from build123d import *

# Parameters (mm, degrees)
SKETCH1_W           = 60
SKETCH1_H           = 30
BOSS_EXTRUDE1_DEPTH = 10
FILLET1_R           = 4
SHELL1_T            = -2
SKETCH29_W          = 3
SKETCH29_H          = 10
BOSS_EXTRUDE2_DEPTH = 1
SKETCH30_W          = 2
SKETCH30_H          = 10
BOSS_EXTRUDE3_DEPTH = 1
SKETCH31_W          = 1
SKETCH31_H          = 10
BOSS_EXTRUDE4_DEPTH = 1


with BuildPart() as part:
    # Sketch1 → Boss-Extrude1 (new body)
    with BuildSketch(Plane.XY):
        with Locations((8.508287293, 1.740331492)):
            Rectangle(SKETCH1_W, SKETCH1_H)
    extrude(amount=BOSS_EXTRUDE1_DEPTH)

    # Fillet1
    fillet1_edges = [part.edges().sort_by_distance(p)[0] for p in [
        (-21.491712707, 16.740331492, 5),
        (38.508287293, 16.740331492, 5),
        (38.508287293, -13.259668508, 5),
        (-21.491712707, -13.259668508, 5),
    ]]
    fillet(fillet1_edges, radius=FILLET1_R)

    # Shell1
    shell1_openings = [part.faces().sort_by_distance(p)[0] for p in [
        (8.508287293, 1.740331492, 10),
    ]]
    offset(amount=SHELL1_T, openings=shell1_openings, kind=Kind.INTERSECTION)

    # Sketch29 → Boss-Extrude2 (add)
    with BuildSketch(Plane.XY.offset(2)):
        with Locations((22.008287293, 1.740331492)):
            Rectangle(SKETCH29_W, SKETCH29_H)
        with Locations((8.008287293, 1.740331492)):
            Rectangle(SKETCH29_W, SKETCH29_H)
        with Locations((-5.991712707, 1.740331492)):
            Rectangle(SKETCH29_W, SKETCH29_H)
    extrude(amount=BOSS_EXTRUDE2_DEPTH)

    # Sketch30 → Boss-Extrude3 (add)
    with BuildSketch(Plane.XY.offset(3)):
        with Locations((22.008287293, 1.740331492)):
            Rectangle(SKETCH30_W, SKETCH30_H)
        with Locations((8.008287293, 1.740331492)):
            Rectangle(SKETCH30_W, SKETCH30_H)
        with Locations((-5.991712707, 1.740331492)):
            Rectangle(SKETCH30_W, SKETCH30_H)
    extrude(amount=BOSS_EXTRUDE3_DEPTH)

    # Sketch31 → Boss-Extrude4 (add)
    with BuildSketch(Plane.XY.offset(4)):
        with Locations((22.008287293, 1.740331492)):
            Rectangle(SKETCH31_W, SKETCH31_H)
        with Locations((8.008287293, 1.740331492)):
            Rectangle(SKETCH31_W, SKETCH31_H)
        with Locations((-5.991712707, 1.740331492)):
            Rectangle(SKETCH31_W, SKETCH31_H)
    extrude(amount=BOSS_EXTRUDE4_DEPTH)


solid = part.part
The listing builds one solid part. Answer for the finished solid, in the listing's coordinates (mm). A direction names the side the tool comes from. Round coordinates to 2 decimals unless told otherwise and drop trailing zeros. Order: outer loops, then holes, each group sorted by start corner. A loop starts at its lowest first (then second) coordinate and runs counter-clockwise, first axis right, second up. Notation, with made-up numbers: (-1.5, 83.25) - (44.5, 83.25) arc R18 ccw to (44.5, 92.25) - close; hole circle Ø2 at (85.25, 36). An arc over 180 degrees is marked (long way). Write item = value, one per line. Start each with the question number.
1) Section B-B, the plane y = 11.75 is taken. Write down the section's boundary in (x, z), plus the area to 3 significant figures.
2) For a pull along X with two mould halves and no side action, classify faces 3 (the flat face through (36.508, 2, 6)), 4 (the flat face through (-6, -3.26, 3)), 5 (the flat face through (-21.492, 2, 5)), 6 (the flat face through (6, -12, 10)) as released by +X, released by -X, zero draft, split by the parting line, or undercut.
3) Section C-C, the plane x = -12 is taken. Write down the section's boundary in (y, z), plus the area to 3 significant figures.
4) Section A-A, the plane z = 6.75 is taken. Write down the section's boundary in (x, y).
5) For faces 1 (the flat face through (-6, 6.74, 3)), 2 (the flat face through (8, 16.74, 5)), determine the directions among +Z, -Z, +X, -X, +Y, -Y from which every point of the face is accessible in a straight line to the end or side of a thin tool.
6) Given pin 1 (1.1 mm diameter, centred on x = 22, y = -0.5, fed in from +Z); pin 2 (4 mm diameter, centred on x = 15, y = -9, fed in from +Z), each flat-ended and moving along its own axis, determine where each tip first touches the part or whether it passes through.
7) Straight lines are drawn through the part: L1, parallel to X at y = -2.25, z = 4.75; L2, parallel to X at y = 1, z = 3.5; L3, parallel to Y at x = -12.5, z = 7.25. For each, find the intervals that lie inside material, in ascending order.
Results list:
q1.outline = (-21.49, 0) - (38.51, 0) - (38.51, 10) - (36.51, 10) - (36.51, 2) - (-19.49, 2) - (-19.49, 10) - (-21.49, 10) - close
q1.area = 152 mm^2
q2.face_3 = undercut
q2.face_4 = undercut
q2.face_5 = released by -X
q2.face_6 = zero draft
q3.outline = (-13.26, 0) - (16.74, 0) - (16.74, 10) - (14.74, 10) - (14.74, 2) - (-11.26, 2) - (-11.26, 10) - (-13.26, 10) - close
q3.area = 92.0 mm^2
q4.outline = (-21.49, -9.26) arc R4 ccw to (-17.49, -13.26) - (34.51, -13.26) arc R4 ccw to (38.51, -9.26) - (38.51, 12.74) arc R4 ccw to (34.51, 16.74) - (-17.49, 16.74) arc R4 ccw to (-21.49, 12.74) - close; hole (-19.49, -9.26) arc R2 ccw to (-17.49, -11.26) - (34.51, -11.26) arc R2 ccw to (36.51, -9.26) - (36.51, 12.74) arc R2 ccw to (34.51, 14.74) - (-17.49, 14.74) arc R2 ccw to (-19.49, 12.74) - close
q5.face_1 = +Z
q5.face_2 = +Z, -Z, +X, -X, +Y
q6.pin_1 = 5
q6.pin_2 = 2
q7.L1 = -21.49 to -19.49, -6.49 to -5.49, 7.51 to 8.51, 21.51 to 22.51, 36.51 to 38.51
q7.L2 = -21.49 to -19.49, -6.99 to -4.99, 7.01 to 9.01, 21.01 to 23.01, 36.51 to 38.51
q7.L3 = -13.26 to -11.26, 14.74 to 16.74
